Read the model definition and answer for the solid it produces. Units are mm, in the model's axes. A direction names the side the tool comes from. Coordinates: 2 decimals unless noted, no trailing zeros. Loops run counter-clockwise (first coordinate to the right, second up) from the corner with the lowest first, then second, coordinate; pieces in that order, holes last.
from build123d import *

# Parameters (mm, degrees)
F0_R      = 8
F1_DEPTH  = 3
F2_W      = 3
F2_H      = 3
F2_W_2    = 134
F3_DEPTH  = 20
F4_W      = 3
F4_H      = 20
F5_DEPTH  = 134
F6_W      = 126
F6_H      = 3
F7_DEPTH  = 40
F8_R      = 1.5
F9_DEPTH  = 3
F10_R     = 8
F12_DEPTH = 40
F13_R     = 1
F14_DEPTH = 3


with BuildPart() as f1:
    # F0 (on Top) → F1 (new body)
    with BuildSketch(Plane.XY):
        Polygon((-60, 33.034884), (-80, 33.034884), (-80, 18.034884), (-80, 0.034884), (-80, -2.965116), (-80, -17.965116), (-80, -29.965116), (60, -29.965116), (60, -24.965116), (60, -14.965116), (60, -9.965116), (60, -4.965116), (60, 0.034884), (60, 18.034884), (60, 33.034884), (40, 33.034884), (20, 33.034884), (0, 33.034884), (-20, 33.034884), (-40, 33.034884), align=None)
        with Locations((25, -0.468963)):
            Circle(F0_R, mode=Mode.SUBTRACT)
        with Locations((-45, 1.034884)):
            Circle(F0_R, mode=Mode.SUBTRACT)
    extrude(amount=F1_DEPTH)

    # F2 (on face) → F3 (join)
    with BuildSketch(Plane.XY.offset(3)):
        with Locations((-78.5, -28.465116)):
            Rectangle(F2_W, F2_H)
        with Locations((-10, -28.465116)):
            Rectangle(F2_W_2, F2_H)
        Polygon((-80, 30.034884), (-80, -26.965116), (-77, -26.965116), (-77, 33.034884), (-80, 33.034884), align=None)
        with Locations((58.5, -28.465116)):
            Rectangle(F2_W, F2_H)
        Polygon((57, 33.034884), (57, -26.965116), (60, -26.965116), (60, 30.034884), (60, 33.034884), align=None)
    extrude(amount=F3_DEPTH)

    # F4 (on face) → F5 (join)
    with BuildSketch(Plane.YZ.offset(-77)):
        with Locations((28.334884, 13)):
            Rectangle(F4_W, F4_H)
    extrude(amount=F5_DEPTH)

    # F6 (on face) → F7 (cut)
    with BuildSketch(Plane.XY.offset(23)):
        with Locations((-10, 28.334884)):
            Rectangle(F6_W, F6_H)
    extrude(amount=-F7_DEPTH, mode=Mode.SUBTRACT)

    # F8 (on face) → F9 (cut)
    with BuildSketch(Plane(origin=(0, -26.965116, 0), x_dir=(-1, 0, 0), z_dir=(0, 1, 0))):
        with Locations((47, 26.988985)):
            Circle(F8_R)
        with Locations((-27, 26.988985)):
            Circle(F8_R)
        with Locations((10, 26.988985)):
            Circle(F8_R)
    extrude(amount=-F9_DEPTH, mode=Mode.SUBTRACT)

    # F10 (on face) → F12 (cut)
    with BuildSketch(Plane.XY.offset(3)):
        Polygon((53, 26.834884), (-73, 26.834884), (-77, 26.834884), (-77, -26.965116), (57, -26.965116), (57, 26.834884), align=None)
        with Locations((25, -0.468963)):
            Circle(F10_R, mode=Mode.SUBTRACT)
        with Locations((-45, 1.034884)):
            Circle(F10_R, mode=Mode.SUBTRACT)
    extrude(amount=-F12_DEPTH, mode=Mode.SUBTRACT)

    # F13 (on face) → F14 (cut)
    with BuildSketch(Plane.XZ.offset(29.965116)):
        with Locations((-63.899942, 11.5)):
            Circle(F13_R)
        with Locations((-10, 11.5)):
            Circle(F13_R)
        with Locations((42.899329, 11.5)):
            Circle(F13_R)
    extrude(amount=-F14_DEPTH, mode=Mode.SUBTRACT)


solid = f1.part
Item 1: A cutting plane is placed at A-A on y = 16. Determine the outline of the cut face in (x, z).
Numbers:
outline: (-80, 0) - (-77, 0) - (-77, 23) - (-80, 23) - close; (57, 0) - (60, 0) - (60, 23) - (57, 23) - close
Item 2: Determine the mould class of faces 4 (the face through (-9, -26.965, 14)), 5 (the face through (-16, -29, 0)), 6 (the face through (-80, 2, 11)), 7 (the face through (-77, 31, 13)) for opening direction X: released by +X, released by -X, zero draft, split by the parting line, or undercut.
Numbers:
face 4: undercut
face 5: zero draft
face 6: released by -X
face 7: undercut
Item 3: A cutting plane is placed at D-D on z = 15.75. Determine the outline of the cut face in (x, y), then the cut area to 3 significant figures.
Numbers:
outline: (-80, -29.97) - (60, -29.97) - (60, 33.03) - (57, 33.03) - (57, 29.83) - (53, 29.83) - (53, 26.83) - (57, 26.83) - (57, -26.97) - (-77, -26.97) - (-77, 26.83) - (-73, 26.83) - (-73, 29.83) - (-77, 29.83) - (-77, 33.03) - (-80, 33.03) - close
area: 804 mm2
Item 4: A cutting plane is placed at B-B on x = 4. Determine the outline of the cut face in (y, z).
Numbers:
outline: (-29.97, 0) - (-26.97, 0) - (-26.97, 23) - (-29.97, 23) - close; (29.83, 0) - (33.03, 0) - (33.03, 3) - (29.83, 3) - close
Item 5: Which of the six approach directions +Z, -Z, +X, -X, +Y, -Y give full straight-line access (tool end or side, diameter ignored) to faces 1 (the face through (-10, -29, 23)), 2 (the face through (55, 26.835, 11)), 3 (the face through (-75, 29.835, 13))?
Numbers:
face 1: +Z, +X, -X, +Y, -Y
face 2: +Z, -Z
face 3: +Z, +Y
Item 6: Given pin 1 (2.5 mm diameter, centred on x = 15, y = 31, fed in from +Z), flat-ended and moving along its own axis, determine where the tip first touches the part or whether it passes through.
Numbers:
pin 1: stops at z = 3
Item 7: A cutting plane is placed at C-C on z = 1.5. Determine the outline of the cut face in (x, y), then the cut area to 3 significant figures.
Numbers:
outline: (-80, -29.97) - (60, -29.97) - (60, 33.03) - (-80, 33.03) - close; hole (-77, -26.97) - (57, -26.97) - (57, 26.83) - (53, 26.83) - (53, 29.83) - (-73, 29.83) - (-73, 26.83) - (-77, 26.83) - close
area: 1,230 mm2
Item 8: Find the intervals of material crossed by line 1 along X through (y, z) = (-8.5, 1.5); line 2 along Z through (x, y) = (-10, -27.65); line 3 along X through (y, z) = (27.5, 7.5), in increasing order.
Numbers:
line 1: x = -80 to -77, 57 to 60
line 2: z = 0 to 10.5, 12.5 to 23
line 3: x = -80 to -73, 53 to 60
